```python
from build123d import *

# Parameters (mm, degrees)
ESQUISSE8_W        = 69.596
ESQUISSE8_H        = 50.8
BOSS_EXTRU_2_DEPTH = 4
ESQUISSE9_W        = 81.28
ESQUISSE9_H        = 62.48
BOSS_EXTRU_3_DEPTH = 1.5
ESQUISSE10_W       = 5.842
ESQUISSE10_H       = 62.48
BOSS_EXTRU_4_DEPTH = 3.5
ESQUISSE11_W       = 5.834410006
ESQUISSE11_H       = 62.48
BOSS_EXTRU_5_DEPTH = 3.5


with BuildPart() as part:
    # Esquisse8 → Boss.-Extru.2 (new body)
    with BuildSketch(Plane(origin=(0, 0, 0), x_dir=(1, 0, 0), z_dir=(0, 1, 0))):
        with Locations((34.798, 25.4)):
            Rectangle(ESQUISSE8_W, ESQUISSE8_H)
    extrude(amount=BOSS_EXTRU_2_DEPTH)

    # Esquisse9 → Boss.-Extru.3 (add)
    with BuildSketch(Plane(origin=(0, 4, 0), x_dir=(1, 0, 0), z_dir=(0, 1, 0))):
        with Locations((34.798, 25.398)):
            Rectangle(ESQUISSE9_W, ESQUISSE9_H)
    extrude(amount=BOSS_EXTRU_3_DEPTH)

    # Esquisse10 → Boss.-Extru.4 (add)
    with BuildSketch(Plane.XZ.offset(-4)):
        with Locations((-2.921, -25.398)):
            Rectangle(ESQUISSE10_W, ESQUISSE10_H)
    extrude(amount=-BOSS_EXTRU_4_DEPTH)

    # Esquisse11 → Boss.-Extru.5 (add)
    with BuildSketch(Plane(origin=(0, 4, 0), x_dir=(-1, 0, 0), z_dir=(0, -1, 0))):
        with Locations((-72.520794997, 25.398)):
            Rectangle(ESQUISSE11_W, ESQUISSE11_H)
    extrude(amount=-BOSS_EXTRU_5_DEPTH)


solid = part.part
```
Geometry check sheet. Reference: the model listing, model coordinates, mm. A direction names the side the tool comes from. Give positions to 0.01 mm unless a question says otherwise; leave off trailing zeros. Write each loop counter-clockwise with the first axis right and the second up, starting at its lowest first coordinate (ties: lowest second). Pieces come first, ordered by that corner, then holes. Notation, with made-up numbers: (24.5, 78) -> (37.5, 78) arc R14 cw to (37.5, 94) -> close; hole circle Ø1 at (-14.5, 11.25). An arc over 180 degrees is marked (long way). One line per question, with ' | ' between items.
Item 1: Sectioned sample at C-C, the plane y = 1.5. Record the boundary of the cut face in (x, z), plus the area to 3 significant figures.
Determined:
outline: (0, -50.8) -> (69.6, -50.8) -> (69.6, 0) -> (0, 0) -> close | area: 3,540 mm^2
Item 2: Sectioned sample at B-B, the plane z = -15.5. Record the boundary of the cut face in (x, y), plus the area to 3 significant figures.
Determined:
outline: (-5.84, 4) -> (0, 4) -> (0, 0) -> (69.6, 0) -> (69.6, 4) -> (75.44, 4) -> (75.44, 7.5) -> (69.6, 7.5) -> (69.6, 5.5) -> (0, 5.5) -> (0, 7.5) -> (-5.84, 7.5) -> close | area: 424 mm^2
Item 3: Sectioned sample at A-A, the plane x = 50. Record the boundary of the cut face in (y, z).
Determined:
outline: (0, -50.8) -> (4, -50.8) -> (4, -56.64) -> (5.5, -56.64) -> (5.5, 5.84) -> (4, 5.84) -> (4, 0) -> (0, 0) -> close
Item 4: Scan lines: line 1 along X through (y, z) = (6, -35.5); line 2 along Z through (x, y) = (16.5, 3.75); line 3 along Y through (x, z) = (36, -16.5). Record each from-to range of solid material in increasing order.
Determined:
line 1: -5.84 to 0, 69.6 to 75.44 | line 2: -50.8 to 0 | line 3: 0 to 5.5
Item 5: Depth check by flat-ended pin: pin 1 (8 mm diameter, centred on x = 46, z = -32.5, fed in from +Y); pin 2 (3 mm diameter, centred on y = 1, z = -33, fed in from +X); pin 3 (3 mm diameter, centred on x = 18.5, y = 2, fed in from +Z). Enter the tip coordinate at first touch or a pass-through.
Determined:
pin 1: y = 5.5 | pin 2: x = 69.6 | pin 3: z = 0
Item 6: Access from +Z, -Z, +X, -X, +Y, -Y to the whole of each face (thin tool, end or side, straight path). Record for faces 1 (the flat face through (0, 2, -25)), 2 (the flat face through (0, 6, -26)), 3 (the flat face through (69.596, 2, -25)).
Determined:
face 1: +Z, -Z, -X, -Y | face 2: +Z, -Z, +Y | face 3: +Z, -Z, +X, -Y
Item 7: Draft check along X on faces 4 (the flat face through (75.438, 6, -25)), 5 (the flat face through (34, 5.5, -26)), 6 (the flat face through (34, 5, 5.842)). Enter one of: released by +X, released by -X, zero draft, split by the parting line, or undercut.
Determined:
face 4: released by +X | face 5: undercut | face 6: zero draft
